Can you work these out from the drawing? Everything is in mm from the part's minimum corner. Round coordinates to 2 decimals unless told otherwise and drop trailing zeros. Order: outer loops, then holes, each group sorted by start corner. A loop starts at its lowest first (then second) coordinate and runs counter-clockwise, first axis right, second up. Notation, with made-up numbers: M 56.5,52.5 L 88.5,52.5 A21 cw 88.5,75.5 Z; hole C 45,37.25 d5. An arc over 180 degrees is marked long. Use one line per item in the form item = value. Start each with the question number.
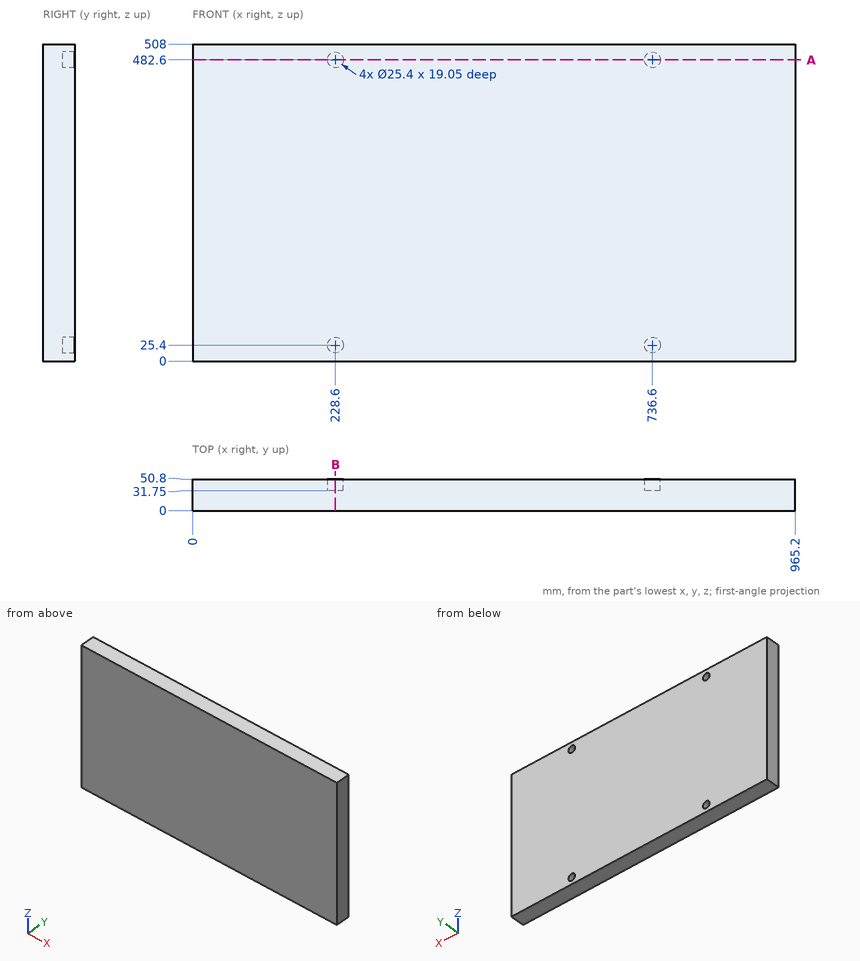
1) Will this pin go through, and if not, where does the flat tip stop? pin 1 Ø20.5 at (x, z) = (736.6, 482.6) entering from +Y.
2) If I drill on line 1 (Z direction, x = 228, y = 42); line 2 (X direction, y = 43, z = 482.6); line 3 (Z direction, x = 742, y = 46), over which ranges is the centre line in solid material (lowest first)?
3) If we section it at A-A on z = 482.6: Write out the boundary of the cut face in (x, y), then the cut area to 3 significant figures.
4) If we section it at B-B on x = 228.6: Write out the boundary of the cut face in (y, z).
Completed:
q1.pin_1 = 31.75
q2.line_1 = 0 to 12.71, 38.09 to 469.91, 495.29 to 508
q2.line_2 = 0 to 215.9, 241.3 to 723.9, 749.3 to 965.2
q2.line_3 = 0 to 13.91, 36.89 to 471.11, 494.09 to 508
q3.outline = M 0,0 L 965.2,0 L 965.2,50.8 L 749.3,50.8 L 749.3,31.75 L 723.9,31.75 L 723.9,50.8 L 241.3,50.8 L 241.3,31.75 L 215.9,31.75 L 215.9,50.8 L 0,50.8 Z
q3.area = 48,100 mm²
q4.outline = M 0,0 L 50.8,0 L 50.8,12.7 L 31.75,12.7 L 31.75,38.1 L 50.8,38.1 L 50.8,469.9 L 31.75,469.9 L 31.75,495.3 L 50.8,495.3 L 50.8,508 L 0,508 Z
